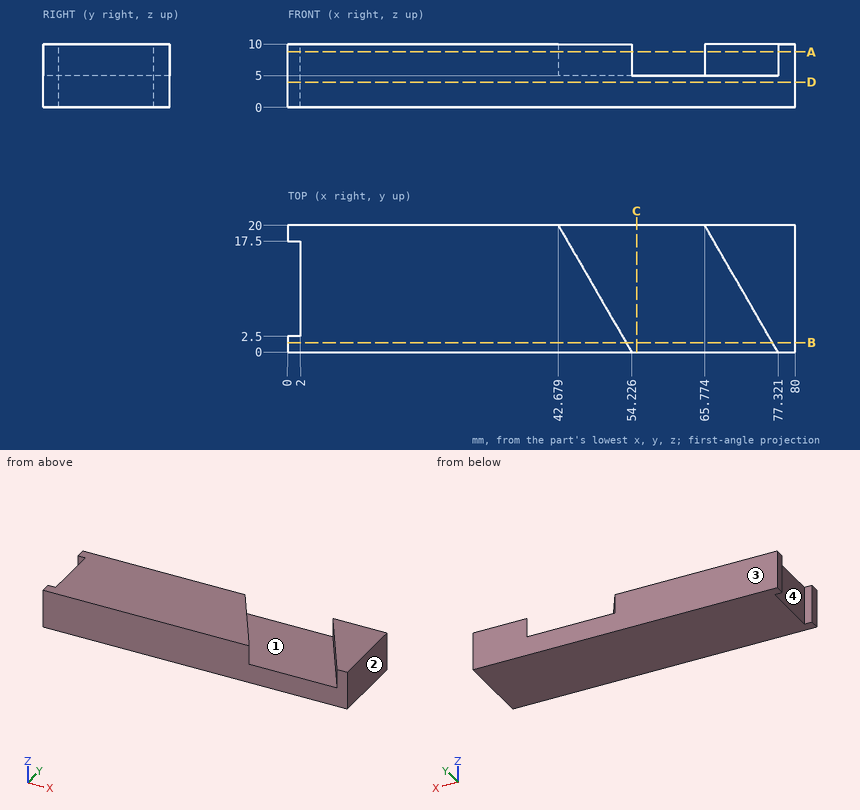
Design review of the part shown in the three views and the two pictorial views. Dimensions are in mm from the part's minimum x, y and z. Give positions to 0.01 mm unless a question says otherwise; leave off trailing zeros. Loops run counter-clockwise (first coordinate to the right, second up) from the corner with the lowest first, then second, coordinate; pieces in that order, holes last. Notation, with made-up numbers: (2, 33.25) -> (20, 33.25) arc R8 ccw to (20, 39.25) -> close; hole circle Ø8 at (72.25, 27.25). An arc over 180 degrees is marked (long way). Answer as a JSON object with one key per item and string values. Group by question number.
Q1. Take a section at D-D (z = 4). Write out the cut boundary in (x, y).
Q2. Draft analysis for pull direction X (two halves, no side actions). For the marked faces 1, 2, 3 and 4, state which applies: pulls with the +X half, pulls with the -X half, needs draft (parallel to the pull), parting line crosses it, or undercut.
Q3. Wall thickness on line 1 along X through (y, z) = (13.75, 4.5); line 2 along Z through (x, y) = (68.5, 4.5); line 3 along X through (y, z) = (8.75, 8.25) (1 decimal): over which ranges is each line inside the solid? List them lowest first.
Q4. Insertion check: pin 1 (3 mm diameter, centred on y = 7.5, z = 8.5, fed in from -X); pin 2 (1 mm diameter, centred on x = 55, y = 2, fed in from +Z). Each pin has a flat end and moves straight along its axis. Give the tip position at first contact, or say it passes through.
Q5. Take a section at C-C (x = 55). Write out the cut boundary in (y, z), plus the area to 3 significant figures.
Q6. Take a section at B-B (y = 1.5). Write out the cut boundary in (x, z) (1 decimal).
Q7. Take a section at A-A (z = 8.75). Write out the cut boundary in (x, y), plus the area to 3 significant figures.
Answer below:
{
 "1": {"outline": "(0, 0) -> (80, 0) -> (80, 20) -> (0, 20) -> (0, 17.5) -> (2, 17.5) -> (2, 2.5) -> (0, 2.5) -> close"},
 "2": {"face 1": "undercut", "face 2": "pulls with the +X half", "face 3": "needs draft", "face 4": "pulls with the -X half"},
 "3": {"line 1": "x = 2 to 80", "line 2": "z = 0 to 5", "line 3": "x = 2 to 49.2, 72.3 to 80"},
 "4": {"pin 1": "stops at x = 2", "pin 2": "stops at z = 5"},
 "5": {"outline": "(0, 0) -> (20, 0) -> (20, 5) -> (0, 5) -> close", "area": "100 mm2"},
 "6": {"outline": "(0, 0) -> (80, 0) -> (80, 10) -> (76.5, 10) -> (76.5, 5) -> (53.4, 5) -> (53.4, 10) -> (0, 10) -> close"},
 "7": {"outline": "(0, 0) -> (54.23, 0) -> (42.68, 20) -> (0, 20) -> (0, 17.5) -> (2, 17.5) -> (2, 2.5) -> (0, 2.5) -> close; (65.77, 20) -> (77.32, 0) -> (80, 0) -> (80, 20) -> close", "area": "1,110 mm2"}
}
